Drawing for the job (mm, zero at the part's lowest x, y, z). Round coordinates to 2 decimals unless told otherwise and drop trailing zeros. Loops run counter-clockwise (first coordinate to the right, second up) from the corner with the lowest first, then second, coordinate; pieces in that order, holes last. Notation, with made-up numbers: M 88.25,51 L 140.25,51 A17 cw 140.25,76 Z; hole C -17.75,-11 d9. An arc over 180 degrees is marked long. Write each question's results on one line, items separated by ' | '.
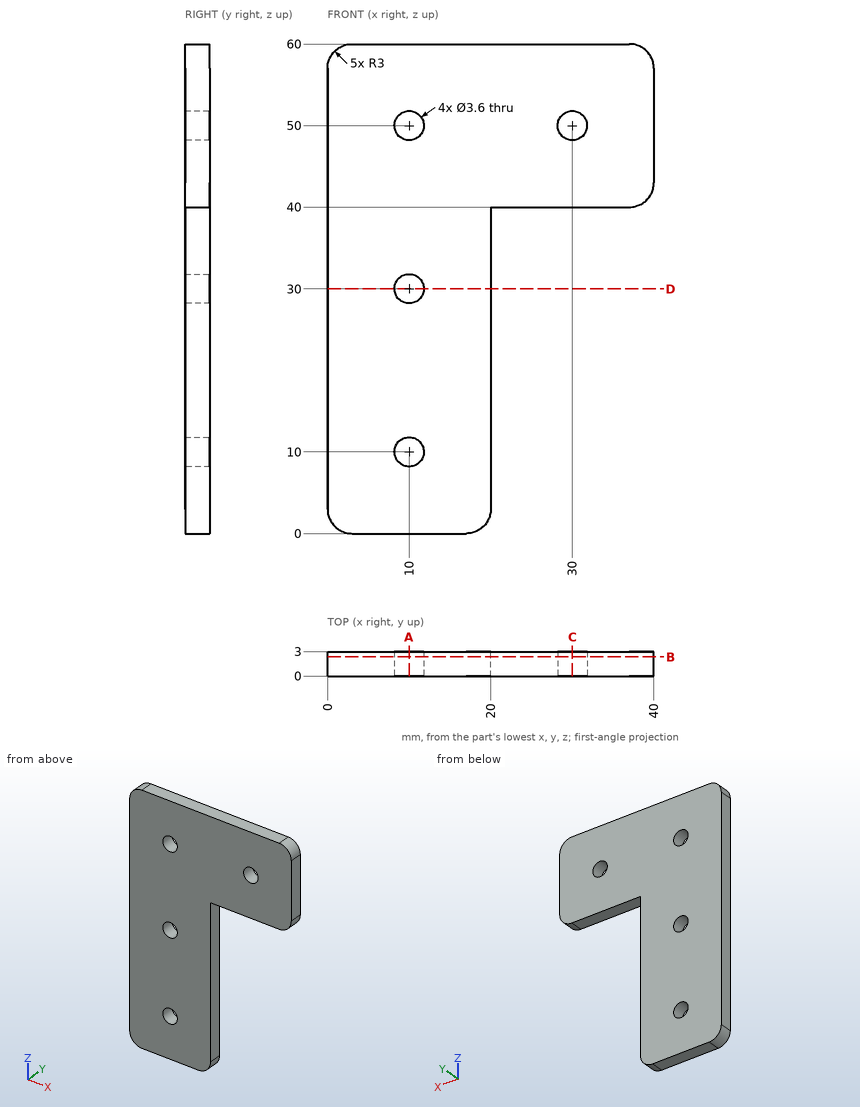
Item 1: Wall check: L1, parallel to X at y = 1.85, z = 50; L2, parallel to X at y = 1.15, z = 10; L3, parallel to Z at x = 11, y = 2. Give the ranges that are in metal, low to high.
Filled sheet:
L1: 0 to 8.2, 11.8 to 28.2, 31.8 to 40 | L2: 0 to 8.2, 11.8 to 20 | L3: 0 to 8.5, 11.5 to 28.5, 31.5 to 48.5, 51.5 to 60
Item 2: Band-saw the part on C-C on x = 30. Give the cut face in (y, z), and give its area (3 significant figures).
Filled sheet:
outline: M 0,40 L 3,40 L 3,48.2 L 0,48.2 Z; M 0,51.8 L 3,51.8 L 3,60 L 0,60 Z | area: 49.2 mm^2
Item 3: Band-saw the part on A-A on x = 10. Give the cut face in (y, z).
Filled sheet:
outline: M 0,0 L 3,0 L 3,8.2 L 0,8.2 Z; M 0,11.8 L 3,11.8 L 3,28.2 L 0,28.2 Z; M 0,31.8 L 3,31.8 L 3,48.2 L 0,48.2 Z; M 0,51.8 L 3,51.8 L 3,60 L 0,60 Z
Item 4: Band-saw the part on D-D on z = 30. Give the cut face in (x, y), and give its area (3 significant figures).
Filled sheet:
outline: M 0,0 L 8.2,0 L 8.2,3 L 0,3 Z; M 11.8,0 L 20,0 L 20,3 L 11.8,3 Z | area: 49.2 mm^2
Item 5: Band-saw the part on B-B on y = 2.35. Give the cut face in (x, z), and give its area (3 significant figures).
Filled sheet:
outline: M 0,3 A3 ccw 3,0 L 17,0 A3 ccw 20,3 L 20,40 L 37,40 A3 ccw 40,43 L 40,57 A3 ccw 37,60 L 3,60 A3 ccw 0,57 Z; hole C 10,10 d3.6; hole C 10,30 d3.6; hole C 10,50 d3.6; hole C 30,50 d3.6 | area: 1,550 mm^2
Item 6: Drop flat-ended pins along their axis: P1, Ø2, axis at x = 30, z = 50, coming from the -Y side; P2, Ø4.5, axis at x = 10, z = 50, coming from the -Y side; P3, Ø0.9, axis at y = 1, z = 24, coming from the +X side. Give the stop position or say it passes through.
Filled sheet:
P1: through | P2: y = 0 | P3: x = 20
